Here's how the part is built. I have some questions about the finished solid (model axes, mm). Face numbers are marked on the shaded views. A direction names the side the tool comes from. Give positions to 0.01 mm unless a question says otherwise; leave off trailing zeros. Order: outer loops, then holes, each group sorted by start corner. A loop starts at its lowest first (then second) coordinate and runs counter-clockwise, first axis right, second up.
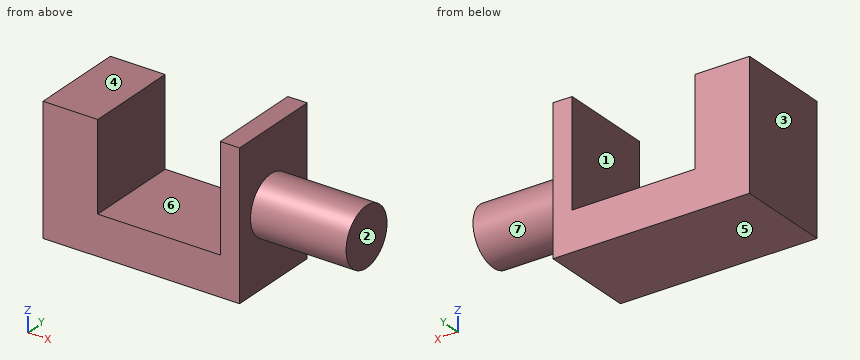
from build123d import *

# Parameters (mm, degrees)
F1_DEPTH = 25.4
F2_R     = 7.699785
F3_DEPTH = 25.4


with BuildPart() as f1:
    # F0 (on Front) → F1 (new body)
    with BuildSketch(Plane.XZ):
        Polygon((0, 33.744156), (0, 0), (52.241661, 0), (52.241661, 38.369093), (47.122207, 38.369093), (47.122207, 10.425531), (14.543891, 10.425531), (14.543891, 33.744156), align=None)
    extrude(amount=F1_DEPTH)

    # F2 (on face) → F3 (join)
    with BuildSketch(Plane.YZ.offset(52.241661)):
        with Locations((-13.601066, 19.184543)):
            Circle(F2_R)
    extrude(amount=F3_DEPTH)


solid = f1.part
Q1. If we section it at B-B on y = -4.25: List the corners of the cut face in (x, z) for me.
Filled sheet:
outline: (0, 0) - (52.24, 0) - (52.24, 38.37) - (47.12, 38.37) - (47.12, 10.43) - (14.54, 10.43) - (14.54, 33.74) - (0, 33.74) - close
Q2. If we section it at D-D on z = 22: List the corners of the cut face in (x, y) for me, plus the area to 3 significant figures.
Filled sheet:
outline: (0, -25.4) - (14.54, -25.4) - (14.54, 0) - (0, 0) - close; (47.12, -25.4) - (52.24, -25.4) - (52.24, -20.77) - (77.64, -20.77) - (77.64, -6.43) - (52.24, -6.43) - (52.24, 0) - (47.12, 0) - close
area: 864 mm2
Q3. I need wall thicknesses on L1, parallel to X at y = -13.5, z = 28; L2, parallel to X at y = -15.75, z = 21.5; L3, parallel to Z at x = 26.5, y = -21.5. Which ranges of each line are inside material? Lowest first, please.
Filled sheet:
L1: x = 0 to 14.54, 47.12 to 52.24
L2: x = 0 to 14.54, 47.12 to 77.64
L3: z = 0 to 10.43
Q4. I'm going to push flat-ended pins straight in: P1, Ø1, axis at x = 69, y = -12, coming from the -Z side; P2, Ø7.5, axis at x = 35, y = -13.5, coming from the +Z side; P3, Ø12, axis at x = 31, z = 20.5, coming from the +Y side; P4, Ø11.5, axis at x = 8, y = -13.5, coming from the +Z side. Where does each tip first touch, or does it pass through?
Filled sheet:
P1: stops at z = 11.56
P2: stops at z = 10.43
P3: passes through
P4: stops at z = 33.74
Q5. Thinking about a two-plate mould opening in X: for the marked faces 1, 2 and 3, which applies, released by +X, released by -X, zero draft, split by the parting line, or undercut?
Filled sheet:
face 1: undercut
face 2: released by +X
face 3: released by -X
Q6. If we section it at C-C on x = 8.5: List the corners of the cut face in (y, z) for me.
Filled sheet:
outline: (-25.4, 0) - (0, 0) - (0, 33.74) - (-25.4, 33.74) - close
Q7. If we section it at A-A on z = 29: List the corners of the cut face in (x, y) for me.
Filled sheet:
outline: (0, -25.4) - (14.54, -25.4) - (14.54, 0) - (0, 0) - close; (47.12, -25.4) - (52.24, -25.4) - (52.24, 0) - (47.12, 0) - close
Q8. For the marked faces 4, 5, 6 and 7, which set-ups out of +Z, -Z, +X, -X, +Y, -Y let a thin tool reach every point of the face, with its end or its side?
Filled sheet:
face 4: +Z, -X, +Y, -Y
face 5: -Z, +X, -X, +Y, -Y
face 6: +Z, +Y, -Y
face 7: +X
